```python
from build123d import *

# Parameters (mm, degrees)
SKETCH1_R           = 12.5
BOSS_EXTRUDE1_DEPTH = 43
SKETCH2_R           = 3.5
BOSS_EXTRUDE2_DEPTH = 2.38
SKETCH3_R           = 1.25
CUT_EXTRUDE1_DEPTH  = 4


with BuildPart() as part:
    # Sketch1 → Boss-Extrude1 (new body)
    with BuildSketch(Plane(origin=(0, 0, 0), x_dir=(1, 0, 0), z_dir=(0, 1, 0))):
        Circle(SKETCH1_R)
    extrude(amount=BOSS_EXTRUDE1_DEPTH)

    # Sketch2 → Boss-Extrude2 (add)
    with BuildSketch(Plane(origin=(0, 43, 0), x_dir=(1, 0, 0), z_dir=(0, 1, 0))):
        Circle(SKETCH2_R)
    extrude(amount=BOSS_EXTRUDE2_DEPTH)

    # Sketch3 → Cut-Extrude1 (cut)
    with BuildSketch(Plane(origin=(0, 43, 0), x_dir=(1, 0, 0), z_dir=(0, 1, 0))):
        with Locations((0, 8.5)):
            Circle(SKETCH3_R)
        with Locations((0, -8.5)):
            Circle(SKETCH3_R)
    extrude(amount=-CUT_EXTRUDE1_DEPTH, mode=Mode.SUBTRACT)


solid = part.part
```
For this review, take the finished solid that the model builds, in its own axes (mm). A direction names the side the tool comes from. Round coordinates to 2 decimals unless told otherwise and drop trailing zeros. Write each loop counter-clockwise with the first axis right and the second up, starting at its lowest first coordinate (ties: lowest second). Pieces come first, ordered by that corner, then holes. Notation, with made-up numbers: (73, 76.25) -> (128, 76.25) arc R29 cw to (128, 115.25) -> close; hole circle Ø4 at (49, 64). An arc over 180 degrees is marked (long way). One line per question, with ' | ' between items. Start each with the question number.
1) Add section C-C (y = 41.5). Write out the cut boundary in (x, z), and give its area (3 significant figures).
2) For pin 1 Ø12 at (y, z) = (36.5, 1) entering from -X; pin 2 Ø1.5 at (x, z) = (9.5, 0.5) entering from +Y; pin 3 Ø1.2 at (x, z) = (0, -9) entering from +Y; pin 4 Ø3 at (x, y) = (-6.5, 35.5) entering from -Z, all flat-tipped, find the tip position at first contact; note any pin that passes through.
3) Add section D-D (y = 28). Write out the cut boundary in (x, z), and give its area (3 significant figures).
4) Machinability: for faces 1 (the cylindrical face through (3.233, 44.173, 1.341)), 2 (the flat face through (0, 45.38, 0)), which of the approach directions +Z, -Z, +X, -X, +Y, -Y give a long, thin tool a straight path to every point of the face, cutting with its end or side? Answer none if there is none.
5) Wall thickness on line 1 along Z through (x, y) = (0, 41.8); line 2 along Y through (x, z) = (3.25, -8.75); line 3 along X through (y, z) = (42, -8.5): over which ranges is each line inside the solid? List them lowest first.
6) Add section B-B (z = 0). Write out the cut boundary in (x, y).
7) Add section A-A (x = 0). Write out the cut boundary in (y, z).
8) Mouldability with a two-part tool opening along X and no side actions: class faces 3 (the cylindrical face through (11.923, 21.199, -3.755)), 4 (the flat face through (0, 0, 0)), 5 (the cylindrical face through (0.672, 41.028, -9.554)), 6 (the cylindrical face through (-0.27, 41.03, 9.72)) as +X half, -X half, draft (parallel to the pull), parting line (faces both ways), or undercut.
Reported:
1) outline: circle Ø25 at (0, 0); hole circle Ø2.5 at (0, -8.5); hole circle Ø2.5 at (0, 8.5) | area: 481 mm²
2) pin 1: stops at x = -12.5 | pin 2: stops at y = 43 | pin 3: stops at y = 39 | pin 4: stops at z = -11.46
3) outline: circle Ø25 at (0, 0) | area: 491 mm²
4) face 1: +Y | face 2: +Z, -Z, +X, -X, +Y
5) line 1: z = -12.5 to -9.75, -7.25 to 7.25, 9.75 to 12.5 | line 2: y = 0 to 43 | line 3: x = -9.17 to -1.25, 1.25 to 9.17
6) outline: (-12.5, 0) -> (12.5, 0) -> (12.5, 43) -> (3.5, 43) -> (3.5, 45.38) -> (-3.5, 45.38) -> (-3.5, 43) -> (-12.5, 43) -> close
7) outline: (0, -12.5) -> (43, -12.5) -> (43, -9.75) -> (39, -9.75) -> (39, -7.25) -> (43, -7.25) -> (43, -3.5) -> (45.38, -3.5) -> (45.38, 3.5) -> (43, 3.5) -> (43, 7.25) -> (39, 7.25) -> (39, 9.75) -> (43, 9.75) -> (43, 12.5) -> (0, 12.5) -> close
8) face 3: parting line | face 4: draft | face 5: undercut | face 6: undercut
